```python
from build123d import *

# Parameters (mm, degrees)
SKETCH1_R           = 1.5
SKETCH1_R_2         = 0.75
BOSS_EXTRUDE1_DEPTH = 2
SKETCH1_3_W         = 10
SKETCH1_3_H         = 5
BOSS_EXTRUDE2_DEPTH = 1
SKETCH1_4_R         = 0.75
CUT_EXTRUDE1_DEPTH  = 1
SKETCH1_5_W         = 10
SKETCH1_5_H         = 5
SKETCH1_5_W_2       = 8
SKETCH1_5_H_2       = 3
SKETCH1_5_R         = 1
BOSS_EXTRUDE3_DEPTH = 5


with BuildPart() as part:
    # Sketch1 → Boss-Extrude1 (new body)
    with BuildSketch(Plane(origin=(0, 0, 0), x_dir=(1, 0, 0), z_dir=(0, 1, 0))):
        with Locations(Location((-2.5, 0, 0), (0, 0, 270))):
            Circle(SKETCH1_R)
        with Locations((-2.5, 0)):
            Circle(SKETCH1_R_2, mode=Mode.SUBTRACT)
        with Locations((-2.5, 0)):
            Circle(SKETCH1_R_2)
        with Locations(Location((2.5, 0, 0), (0, 0, 270))):
            Circle(SKETCH1_R)
        with Locations((2.5, 0)):
            Circle(SKETCH1_R_2, mode=Mode.SUBTRACT)
        with Locations((2.5, 0)):
            Circle(SKETCH1_R_2)
    extrude(amount=BOSS_EXTRUDE1_DEPTH)

    # Sketch1_3 → Boss-Extrude2 (add)
    with BuildSketch(Plane(origin=(0, 0, 0), x_dir=(1, 0, 0), z_dir=(0, 1, 0))):
        Rectangle(SKETCH1_3_W, SKETCH1_3_H)
    extrude(amount=BOSS_EXTRUDE2_DEPTH)

    # Sketch1_4 → Cut-Extrude1 (cut)
    with BuildSketch(Plane(origin=(0, 0, 0), x_dir=(1, 0, 0), z_dir=(0, 1, 0))):
        with Locations(Location((-2.5, 0, 0), (0, 0, 270))):
            Circle(SKETCH1_4_R)
        with Locations(Location((2.5, 0, 0), (0, 0, 270))):
            Circle(SKETCH1_4_R)
    extrude(amount=CUT_EXTRUDE1_DEPTH, mode=Mode.SUBTRACT)

    # Sketch1_5 → Boss-Extrude3 (add)
    with BuildSketch(Plane(origin=(0, 0, 0), x_dir=(1, 0, 0), z_dir=(0, 1, 0))):
        Rectangle(SKETCH1_5_W, SKETCH1_5_H)
        Rectangle(SKETCH1_5_W_2, SKETCH1_5_H_2, mode=Mode.SUBTRACT)
        with Locations(Location((0, 0, 0), (0, 0, 270))):
            Circle(SKETCH1_5_R)
    extrude(amount=-BOSS_EXTRUDE3_DEPTH)


solid = part.part
```
Verification items for the finished model (mm, model axes). A direction names the side the tool comes from. Coordinates: 2 decimals unless noted, no trailing zeros. Order: outer loops, then holes, each group sorted by start corner. A loop starts at its lowest first (then second) coordinate and runs counter-clockwise, first axis right, second up. Notation, with made-up numbers: (59.5, 15) -> (113.5, 15) arc R28 ccw to (113.5, 44) -> close; hole circle Ø3 at (-25, 31). An arc over 180 degrees is marked (long way). Put each result on its own line as item: value. Start each with the question number.
1) Cross-section at C-C (x = 0). Enter the section's corners in (y, z), plus the area to 3 significant figures.
2) Release check for a two-part mould opening along X. For faces 4 (the flat face through (0, -2, 1.5)), 5 (the flat face through (0, -2, -2.5)), 6 (the flat face through (5, -2, 0)) record: pulls with the +X half, pulls with the -X half, needs draft (parallel to the pull), parting line crosses it, or undercut.
3) Go/stop test with a flat-tipped pin: pin 1 (1.6 mm diameter, centred on x = 2.5, z = 0.5, fed in from -Y). Record where the tip stops, or that it passes through.
4) Tool access check on faces 1 (the cylindrical face through (-3.83, 1.49, 0.69)), 2 (the flat face through (0, -5, -2)), 3 (the flat face through (-4, -2, 0)). Record the directions out of +Z, -Z, +X, -X, +Y, -Y that give a thin tool (end or side, any length) a straight path to the whole face; none if there is none.
5) Cross-section at A-A (y = -3.5). Enter the section's corners in (x, z), plus the area to 3 significant figures.
6) Material ranges on L1, parallel to X at y = 0.65, z = 0; L2, parallel to Z at x = -1.5, y = -3; L3, parallel to Z at x = -0.75, y = -3, recorded low to high.
7) Cross-section at D-D (y = 1.25). Enter the section's corners in (x, z).
8) Cross-section at B-B (z = 0). Enter the section's corners in (x, y), plus the area to 3 significant figures.
Geometry check:
1. outline: (-5, -2.5) -> (1, -2.5) -> (1, 2.5) -> (-5, 2.5) -> (-5, 1.5) -> (0, 1.5) -> (0, 1) -> (-5, 1) -> (-5, -1) -> (0, -1) -> (0, -1.5) -> (-5, -1.5) -> close
1. area: 25.0 mm^2
2. face 4: undercut
2. face 5: needs draft
2. face 6: pulls with the +X half
3. pin 1: stops at y = 0
4. face 1: +Y
4. face 2: +Z, -Z, +X, -X, -Y
4. face 3: -Y
5. outline: (-5, -2.5) -> (5, -2.5) -> (5, 2.5) -> (-5, 2.5) -> close; circle Ø2 at (0, 0); hole (-4, -1.5) -> (4, -1.5) -> (4, 1.5) -> (-4, 1.5) -> close
5. area: 29.1 mm^2
6. L1: x = -5 to -3.25, -1.75 to 1.75, 3.25 to 5
6. L2: z = -2.5 to -1.5, 1.5 to 2.5
6. L3: z = -2.5 to -1.5, -0.66 to 0.66, 1.5 to 2.5
7. outline: circle Ø3 at (-2.5, 0); circle Ø3 at (2.5, 0)
8. outline: (-5, -5) -> (-4, -5) -> (-4, 0) -> (-3.25, 0) -> (-3.25, 1) -> (-1.75, 1) -> (-1.75, 0) -> (-1, 0) -> (-1, -5) -> (1, -5) -> (1, 0) -> (1.75, 0) -> (1.75, 1) -> (3.25, 1) -> (3.25, 0) -> (4, 0) -> (4, -5) -> (5, -5) -> (5, 1) -> (4, 1) -> (4, 2) -> (1, 2) -> (1, 1) -> (-1, 1) -> (-1, 2) -> (-4, 2) -> (-4, 1) -> (-5, 1) -> close
8. area: 33.0 mm^2
